```python
from build123d import *

# Parameters (mm, degrees)
BOSS_EXTRUDE1_DEPTH = 6.35
SKETCH2_R           = 2.54
BOSS_EXTRUDE2_DEPTH = 38.1
SKETCH3_R           = 2.54
CUT_EXTRUDE1_DEPTH  = 38.1


with BuildPart() as part:
    # Sketch1 → Boss-Extrude1 (new body)
    with BuildSketch(Plane.XY):
        with BuildLine():
            Line((8.255, 0), (8.255, -37.839819965))
            ThreePointArc((8.255, -37.839819965), (4.8895, -41.623801962), (0.738716667, -38.722749098))
            Line((0.738716667, -38.722749098), (-8.030280556, -1.91301312))
            ThreePointArc((-8.030280556, -1.91301312), (-0.963083333, 8.198627659), (8.255, 0))
        make_face()
    extrude(amount=BOSS_EXTRUDE1_DEPTH)

    # Sketch2 → Boss-Extrude2 (add)
    with BuildSketch(Plane(origin=(0, 0, 0), x_dir=(-1, 0, 0), z_dir=(0, 0, -1))):
        with Locations((-4.445, -37.839819965)):
            Circle(SKETCH2_R)
    extrude(amount=BOSS_EXTRUDE2_DEPTH)

    # Sketch3 → Cut-Extrude1 (cut)
    with BuildSketch(Plane.XY.offset(6.35)):
        Circle(SKETCH3_R)
    extrude(amount=-CUT_EXTRUDE1_DEPTH, mode=Mode.SUBTRACT)


solid = part.part
```
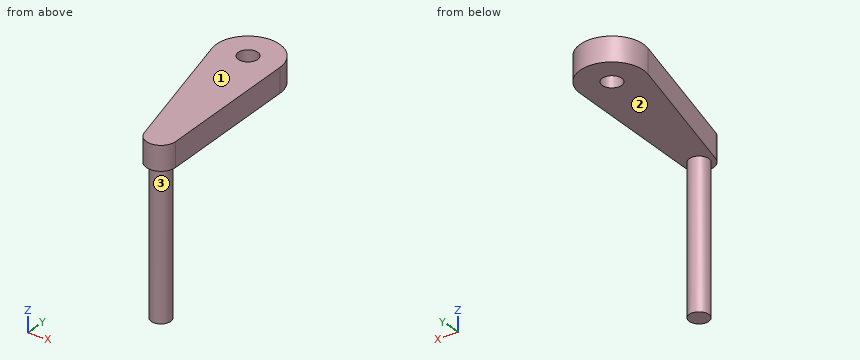
Work out the finished part from the listing and answer in its coordinate system (mm). Face numbers are marked on the shaded views. Coordinates: 2 decimals unless noted, no trailing zeros. Write each loop counter-clockwise with the first axis right and the second up, starting at its lowest first coordinate (ties: lowest second). Pieces come first, ordered by that corner, then holes.
Q1. Find the intervals of material crossed by line 1 (Z direction, x = -2, y = -16.5); line 2 (X direction, y = -21, z = 4) (3 decimals); line 3 (X direction, y = -38.5, z = -11.5), in increasing order.
Q2. Determine the mould class of the marked faces 1, 2 and 3 for opening direction Z: released by +Z, released by -Z, zero draft, split by the parting line, or undercut.
Q3. A cutting plane is placed at D-D, the plane z = -21. Give the vertices of the cut face in (x, y) (3 decimals), then the cut area to 3 significant figures.
Q4. A cutting plane is placed at B-B, the plane x = 0. Give the vertices of the cut face in (y, z) (3 decimals), then the cut area to 3 significant figures.
Q5. A cutting plane is placed at C-C, the plane y = -12.5. Give the vertices of the cut face in (x, z) (3 decimals).
Q6. A cutting plane is placed at A-A, the plane z = 1. Give the vertices of the cut face in (x, y) (3 decimals), then the cut area to 3 significant figures.
Q7. Each of these flat-tipped pins is pushed along its axis until it touches: pin 1 Ø4 at (x, z) = (4, 1.5) entering from +Y; pin 2 Ø8.5 at (x, y) = (-3, -11) entering from -Z. Where does it stop, or does it pass through?
Findings below:
1. line 1: z = 0 to 6.35
1. line 2: x = -3.483 to 8.255
1. line 3: x = 1.99 to 6.9
2. face 1: released by +Z
2. face 2: released by -Z
2. face 3: zero draft
3. outline: circle Ø5.08 at (4.445, -37.84)
3. area: 20.3 mm2
4. outline: (-35.622, 0) - (-2.54, 0) - (-2.54, 6.35) - (-35.622, 6.35) - close; (2.54, 0) - (8.255, 0) - (8.255, 6.35) - (2.54, 6.35) - close
4. area: 246 mm2
5. outline: (-5.508, 0) - (8.255, 0) - (8.255, 6.35) - (-5.508, 6.35) - close
6. outline: (-8.03, -1.913) - (0.739, -38.723) arc R3.81 ccw to (8.255, -37.84) - (8.255, 0) arc R8.255 ccw (long way) to start; hole circle Ø5.08 at (0, 0)
6. area: 572 mm2
7. pin 1: stops at y = 8.01
7. pin 2: stops at z = 0
